from build123d import *

# Parameters (mm, degrees)
SKETCH2_R               = 10
BOSS_EXTRUDE1_DEPTH     = 12
SKETCH3_R               = 17.65
CUT_EXTRUDE1_DEPTH      = 3
CUT_EXTRUDE2_DEPTH      = 114
CUT_EXTRUDE2_DEPTH_BACK = 114
SKETCH5_R               = 3
CUT_EXTRUDE3_DEPTH      = 114
SKETCH6_R               = 16
CUT_EXTRUDE4_DEPTH      = 113.720894248
SKETCH7_W               = 51
SKETCH7_H               = 43
CUT_EXTRUDE5_DEPTH      = 2
CHAMFER1_SIZE           = 2
CUT_EXTRUDE6_DEPTH      = 8
CUT_EXTRUDE7_DEPTH      = 3
CUT_EXTRUDE8_DEPTH      = 113.720894248
SKETCH11_R              = 3
BOSS_EXTRUDE2_DEPTH     = 12
FILLET1_R               = 6
CUT_EXTRUDE9_DEPTH      = 10


with BuildPart() as part:
    # Sketch2 → Boss-Extrude1 (new body)
    with BuildSketch(Plane.XY):
        with BuildLine():
            Line((-105, -25), (-105, 25))
            Line((-105, 25), (-5.815477401, 39.574994916))
            ThreePointArc((-5.815477401, 39.574994916), (40, 0), (-5.815477401, -39.574994916))
            Line((-5.815477401, -39.574994916), (-105, -25))
        make_face()
        Circle(SKETCH2_R, mode=Mode.SUBTRACT)
    extrude(amount=BOSS_EXTRUDE1_DEPTH)

    # Sketch3 → Cut-Extrude1 (cut)
    with BuildSketch(Plane.XY.offset(12)):
        Circle(SKETCH3_R)
    extrude(amount=-CUT_EXTRUDE1_DEPTH, mode=Mode.SUBTRACT)

    # Sketch4 → Cut-Extrude2 (cut, two sides: drawn at the far end of the back side and taken through both)
    with BuildSketch(Plane.XY.offset(12).offset(-CUT_EXTRUDE2_DEPTH_BACK)):
        with BuildLine():
            Line((-73.3, 7.5), (-81.3, 7.5))
            ThreePointArc((-81.3, 7.5), (-88.8, 0), (-81.3, -7.5))
            Line((-81.3, -7.5), (-73.3, -7.5))
            ThreePointArc((-73.3, -7.5), (-65.8, 0), (-73.3, 7.5))
        make_face()
    extrude(amount=CUT_EXTRUDE2_DEPTH + CUT_EXTRUDE2_DEPTH_BACK, mode=Mode.SUBTRACT)

    # Sketch5 → Cut-Extrude3 (cut, through all)
    with BuildSketch(Plane.XY.offset(12)):
        with Locations((30, 0)):
            Circle(SKETCH5_R)
        with Locations((0, -30)):
            Circle(SKETCH5_R)
        with Locations((-30, 0)):
            Circle(SKETCH5_R)
        with Locations((0, 30)):
            Circle(SKETCH5_R)
    extrude(amount=-CUT_EXTRUDE3_DEPTH, mode=Mode.SUBTRACT)

    # Sketch6 → Cut-Extrude4 (cut, through all)
    with BuildSketch(Plane.XY.offset(9)):
        Circle(SKETCH6_R)
    extrude(amount=-CUT_EXTRUDE4_DEPTH, mode=Mode.SUBTRACT)

    # Sketch7 → Cut-Extrude5 (cut)
    with BuildSketch(Plane(origin=(0, 0, 0), x_dir=(-1, 0, 0), z_dir=(0, 0, -1))):
        with Locations((77.3, 0)):
            Rectangle(SKETCH7_W, SKETCH7_H)
    extrude(amount=-CUT_EXTRUDE5_DEPTH, mode=Mode.SUBTRACT)

    # Chamfer1
    chamfer1_edges = [part.edges().sort_by_distance(p)[0] for p in [
        (-102.8, 21.5, 1),
        (-102.8, -21.5, 1),
        (-51.8, -21.5, 1),
        (-51.8, 21.5, 1),
    ]]
    chamfer(chamfer1_edges, length=CHAMFER1_SIZE)

    # Sketch8 → Cut-Extrude6 (cut)
    with BuildSketch(Plane.XY.offset(12)):
        Polygon((30, -7.505553499), (36.5, -3.75277675), (36.5, 3.75277675), (30, 7.505553499), (23.5, 3.75277675), (23.5, -3.75277675), align=None)
        Polygon((7.505553499, 30), (3.75277675, 36.5), (-3.75277675, 36.5), (-7.505553499, 30), (-3.75277675, 23.5), (3.75277675, 23.5), align=None)
        Polygon((-7.505553499, -30), (-3.75277675, -36.5), (3.75277675, -36.5), (7.505553499, -30), (3.75277675, -23.5), (-3.75277675, -23.5), align=None)
        Polygon((-30, 7.505553499), (-36.5, 3.75277675), (-36.5, -3.75277675), (-30, -7.505553499), (-23.5, -3.75277675), (-23.5, 3.75277675), align=None)
    extrude(amount=-CUT_EXTRUDE6_DEPTH, mode=Mode.SUBTRACT)

    # Sketch9 → Cut-Extrude7 (cut)
    with BuildSketch(Plane.XY.offset(12)):
        with BuildLine():
            Line((-65.8, 12.5), (-57.8, 12.5))
            ThreePointArc((-57.8, 12.5), (-54.8, 15.5), (-57.8, 18.5))
            Line((-57.8, 18.5), (-65.8, 18.5))
            ThreePointArc((-65.8, 18.5), (-68.8, 15.5), (-65.8, 12.5))
        make_face()
        with BuildLine():
            Line((-88.8, 18.5), (-96.8, 18.5))
            ThreePointArc((-96.8, 18.5), (-99.8, 15.5), (-96.8, 12.5))
            Line((-96.8, 12.5), (-88.8, 12.5))
            ThreePointArc((-88.8, 12.5), (-85.8, 15.5), (-88.8, 18.5))
        make_face()
        with BuildLine():
            Line((-59.089545502, -12.5), (-67.089545502, -12.5))
            ThreePointArc((-67.089545502, -12.5), (-70.089545502, -15.5), (-67.089545502, -18.5))
            Line((-67.089545502, -18.5), (-59.089545502, -18.5))
            ThreePointArc((-59.089545502, -18.5), (-56.089545502, -15.5), (-59.089545502, -12.5))
        make_face()
        with BuildLine():
            Line((-88.8, -12.5), (-96.8, -12.5))
            ThreePointArc((-96.8, -12.5), (-99.8, -15.5), (-96.8, -18.5))
            Line((-96.8, -18.5), (-88.8, -18.5))
            ThreePointArc((-88.8, -18.5), (-85.8, -15.5), (-88.8, -12.5))
        make_face()
    extrude(amount=-CUT_EXTRUDE7_DEPTH, mode=Mode.SUBTRACT)

    # Sketch10 → Cut-Extrude8 (cut, through all)
    with BuildSketch(Plane.XY.offset(9)):
        with BuildLine():
            Line((-67.089545502, -13.75), (-59.089545502, -13.75))
            ThreePointArc((-59.089545502, -13.75), (-57.339545502, -15.5), (-59.089545502, -17.25))
            Line((-59.089545502, -17.25), (-67.089545502, -17.25))
            ThreePointArc((-67.089545502, -17.25), (-68.839545502, -15.5), (-67.089545502, -13.75))
        make_face()
        with BuildLine():
            Line((-65.8, 17.25), (-57.8, 17.25))
            ThreePointArc((-57.8, 17.25), (-56.05, 15.5), (-57.8, 13.75))
            Line((-57.8, 13.75), (-65.8, 13.75))
            ThreePointArc((-65.8, 13.75), (-67.55, 15.5), (-65.8, 17.25))
        make_face()
        with BuildLine():
            Line((-96.8, 17.25), (-88.8, 17.25))
            ThreePointArc((-88.8, 17.25), (-87.05, 15.5), (-88.8, 13.75))
            Line((-88.8, 13.75), (-96.8, 13.75))
            ThreePointArc((-96.8, 13.75), (-98.55, 15.5), (-96.8, 17.25))
        make_face()
        with BuildLine():
            Line((-96.8, -13.75), (-88.8, -13.75))
            ThreePointArc((-88.8, -13.75), (-87.05, -15.5), (-88.8, -17.25))
            Line((-88.8, -17.25), (-96.8, -17.25))
            ThreePointArc((-96.8, -17.25), (-98.55, -15.5), (-96.8, -13.75))
        make_face()
    extrude(amount=-CUT_EXTRUDE8_DEPTH, mode=Mode.SUBTRACT)

    # Sketch11 → Boss-Extrude2 (add)
    with BuildSketch(Plane.XY.offset(12)):
        with BuildLine():
            Line((-115, 12.5), (-105, 12.5))
            Line((-105, 12.5), (-105, -12.5))
            Line((-105, -12.5), (-115, -12.5))
            ThreePointArc((-115, -12.5), (-127.5, 0), (-115, 12.5))
        make_face()
        with Locations((-115, 0)):
            Circle(SKETCH11_R, mode=Mode.SUBTRACT)
    extrude(amount=-BOSS_EXTRUDE2_DEPTH)

    # Fillet1
    fillet1_edges = [part.edges().sort_by_distance(p)[0] for p in [
        (-105, -12.5, 6),
        (-105, 12.5, 6),
        (-105, -25, 6),
        (-105, 25, 6),
    ]]
    fillet(fillet1_edges, radius=FILLET1_R)

    # Sketch12 → Cut-Extrude9 (cut)
    with BuildSketch(Plane.XY.offset(12)):
        Polygon((-111.317344252, 6.539983179), (-118.822463699, 6.45926502), (-122.505119447, -0.080718159), (-118.682655748, -6.539983179), (-111.177536301, -6.45926502), (-107.494880553, 0.080718159), align=None)
    extrude(amount=-CUT_EXTRUDE9_DEPTH, mode=Mode.SUBTRACT)


solid = part.part
Verification items for the finished model (mm, model axes). A direction names the side the tool comes from. Coordinates: 2 decimals unless noted, no trailing zeros. Write each loop counter-clockwise with the first axis right and the second up, starting at its lowest first coordinate (ties: lowest second). Pieces come first, ordered by that corner, then holes. Notation, with made-up numbers: M 76.5,60.25 L 121.5,60.25 A25 ccw 121.5,86.25 Z; hole C 42,-12 d2. An arc over 180 degrees is marked long. Use a Markdown table: item, result.
Q1. Sectioned sample at C-C, the plane z = 6.25. Count the separate pieces of the cut face and the enclosed holes in it, plus the area to 3 significant figures.
Reply:
| item | result |
|---|---|
| separate pieces | 1 |
| enclosed holes | 11 |
| area | 7,900 mm² |
Q2. Draft check along X on faces 3 (the face through (-77, 7.5, 7)), 4 (the face through (-43, 1, 12)). Enter one of: +X half, -X half, draft (parallel to the pull), parting line (faces both ways), or undercut.
Reply:
| item | result |
|---|---|
| face 3 | undercut |
| face 4 | draft |
Q3. Go/stop test with flat-tipped pins: P1, Ø0.6, axis at y = 4, z = 1, coming from the -X side; P2, Ø7, axis at x = -115, y = 0, coming from the +Z side; P3, Ø2, axis at x = -112, z = 6.5, coming from the +Y side; P4, Ø3.5, axis at x = -30, y = 0, coming from the -Z side. Record where each tip stops, or that it passes through.
Reply:
| item | result |
|---|---|
| P1 | stops at x = -126.94 |
| P2 | stops at z = 2 |
| P3 | stops at y = 12.5 |
| P4 | passes through |
Q4. Sectioned sample at A-A, the plane x = 0. Record the boundary of the cut face in (y, z), plus the area to 3 significant figures.
Reply:
| item | result |
|---|---|
| outline | M -40,0 L -33,0 L -33,4 L -36.5,4 L -36.5,12 L -40,12 Z; M -27,0 L -16,0 L -16,9 L -17.65,9 L -17.65,12 L -23.5,12 L -23.5,4 L -27,4 Z; M 16,0 L 27,0 L 27,4 L 23.5,4 L 23.5,12 L 17.65,12 L 17.65,9 L 16,9 Z; M 33,0 L 40,0 L 40,12 L 36.5,12 L 36.5,4 L 33,4 Z |
| area | 310 mm² |
Q5. Thickness scan on line 1 (Y direction, x = 0, z = 1.3); line 2 (X direction, y = -2, z = 5.75); line 3 (Y direction, x = 0, z = 11.3). Record the ranges inside material, lowest first.
Reply:
| item | result |
|---|---|
| line 1 | y = -40 to -33, -27 to -16, 16 to 27, 33 to 40 |
| line 2 | x = -127.34 to -121.37, -108.67 to -88.53, -66.07 to -36.5, -23.5 to -15.87, 15.87 to 23.5, 36.5 to 39.95 |
| line 3 | y = -40 to -36.5, -23.5 to -17.65, 17.65 to 23.5, 36.5 to 40 |
Q6. Set-up check for faces 1 (the face through (-93, 12.5, 11)), 2 (the face through (-87.05, -15.46, 5.55)): record each of +Z, -Z, +X, -X, +Y, -Y from which the full face is reachable in a straight line by a thin tool's end or side.
Reply:
| item | result |
|---|---|
| face 1 | +Z |
| face 2 | +Z, -Z |
Q7. Sectioned sample at B-B, the plane x = -113.5. Record the boundary of the cut face in (y, z), plus the area to 3 significant figures.
Reply:
| item | result |
|---|---|
| outline | M -12.5,0 L -2.6,0 L -2.6,2 L -6.48,2 L -6.48,12 L -12.5,12 Z; M 2.6,0 L 12.5,0 L 12.5,12 L 6.52,12 L 6.52,2 L 2.6,2 Z |
| area | 160 mm² |
